Verification items for the finished model (mm, model axes). A direction names the side the tool comes from. Coordinates: 2 decimals unless noted, no trailing zeros. Write each loop counter-clockwise with the first axis right and the second up, starting at its lowest first coordinate (ties: lowest second). Pieces come first, ordered by that corner, then holes. Notation, with made-up numbers: (-22.75, 10) - (-16.75, 10) arc R13 cw to (-16.75, 29) - close; hole circle Ø2 at (2.25, -12.75). An arc over 180 degrees is marked (long way). Answer as CSV lines item,"result". Start each with the question number.
```python
from build123d import *

# Parameters (mm, degrees)
SKETCH1_W           = 90.48
SKETCH1_H           = 132.76
SKETCH1_W_2         = 85.48
SKETCH1_H_2         = 127.76
BOSS_EXTRUDE1_DEPTH = 16
SKETCH2_W           = 90.48
SKETCH2_H           = 132.76
BOSS_EXTRUDE2_DEPTH = 2.5
SKETCH3_R           = 7.5
BOSS_EXTRUDE3_DEPTH = 25
SKETCH4_R           = 7.5
SKETCH4_R_2         = 5
BOSS_EXTRUDE4_DEPTH = 25
SKETCH5_R           = 11
SKETCH5_R_2         = 5
BOSS_EXTRUDE5_DEPTH = 5
SKETCH7_R           = 5
CUT_EXTRUDE2_DEPTH  = 20
CUT_EXTRUDE3_REACH  = 134.76
SKETCH8_R           = 1.75
BOSS_EXTRUDE6_DEPTH = 5
SKETCH10_W          = 65.48
SKETCH10_H          = 107.76
CUT_EXTRUDE4_DEPTH  = 5.25


with BuildPart() as part:
    # Sketch1 → Boss-Extrude1 (new body)
    with BuildSketch(Plane(origin=(0, 0, 0), x_dir=(1, 0, 0), z_dir=(0, 1, 0))):
        Rectangle(SKETCH1_W, SKETCH1_H)
        Rectangle(SKETCH1_W_2, SKETCH1_H_2, mode=Mode.SUBTRACT)
    extrude(amount=BOSS_EXTRUDE1_DEPTH)

    # Sketch2 → Boss-Extrude2 (add)
    with BuildSketch(Plane.XZ):
        Rectangle(SKETCH2_W, SKETCH2_H)
    extrude(amount=BOSS_EXTRUDE2_DEPTH)

    # Sketch3 → Boss-Extrude3 (add)
    with BuildSketch(Plane(origin=(0, 0, -66.38), x_dir=(-1, 0, 0), z_dir=(0, 0, -1))):
        with BuildLine():
            Line((-45.24, 16), (-60, 16))
            ThreePointArc((-60, 16), (-69.25, 6.75), (-60, -2.5))
            Line((-60, -2.5), (-45.24, -2.5))
            Line((-45.24, -2.5), (-45.24, 16))
        make_face()
        with Locations((-60, 6.75)):
            Circle(SKETCH3_R, mode=Mode.SUBTRACT)
    boss_extrude3 = extrude(amount=-BOSS_EXTRUDE3_DEPTH)

    # Mirror1: Boss-Extrude3 across plane
    add(boss_extrude3.mirror(Plane(origin=(0, 0, 0), x_dir=(0, 0, 1), z_dir=(1, 0, 0))))

    # Sketch4 → Boss-Extrude4 (add)
    with BuildSketch(Plane(origin=(0, 0, -66.38), x_dir=(-1, 0, 0), z_dir=(0, 0, -1))):
        with Locations((60, 6.75)):
            Circle(SKETCH4_R)
        with Locations((60, 6.75)):
            Circle(SKETCH4_R_2, mode=Mode.SUBTRACT)
    extrude(amount=-BOSS_EXTRUDE4_DEPTH)

    # Sketch5 → Boss-Extrude5 (add)
    with BuildSketch(Plane(origin=(0, 0, -66.38), x_dir=(-1, 0, 0), z_dir=(0, 0, -1))):
        with Locations((60, 6.75)):
            Circle(SKETCH5_R)
        with Locations((60, 6.75)):
            Circle(SKETCH5_R_2, mode=Mode.SUBTRACT)
    extrude(amount=-BOSS_EXTRUDE5_DEPTH)

    # Sketch7 → Cut-Extrude2 (cut)
    with BuildSketch(Plane.XY.offset(-41.38)):
        with Locations((-60, 6.75)):
            Circle(SKETCH7_R)
        with BuildLine():
            Line((-45.24, -2.5), (-60, -2.5))
            ThreePointArc((-60, -2.5), (-69.25, 6.75), (-60, 16))
            Line((-60, 16), (-45.24, 16))
            Line((-45.24, 16), (-45.24, 8.25))
            Line((-45.24, 8.25), (-54.190524981, 8.25))
            ThreePointArc((-54.190524981, 8.25), (-66, 6.75), (-54.190524981, 5.25))
            Line((-54.190524981, 5.25), (-45.24, 5.25))
            Line((-45.24, 5.25), (-45.24, -2.5))
        make_face()
    extrude(amount=-CUT_EXTRUDE2_DEPTH, mode=Mode.SUBTRACT)

    # Sketch8 → Cut-Extrude3 (cut, up to next)
    with BuildSketch(Plane(origin=(0, 0, -66.38), x_dir=(-1, 0, 0), z_dir=(0, 0, -1)), mode=Mode.PRIVATE) as cut_extrude3_sk1:
        with Locations((60, 14.75)):
            Circle(SKETCH8_R)
    cut_extrude3_tool1 = extrude(cut_extrude3_sk1.sketch, amount=-CUT_EXTRUDE3_REACH, mode=Mode.PRIVATE) & part.part
    add(cut_extrude3_tool1.solids().sort_by_distance((-60, 14.75, -66.38))[0], mode=Mode.SUBTRACT)
    # Sketch8 → Cut-Extrude3 (cut, up to next)
    with BuildSketch(Plane(origin=(0, 0, -66.38), x_dir=(-1, 0, 0), z_dir=(0, 0, -1)), mode=Mode.PRIVATE) as cut_extrude3_sk2:
        with Locations((68, 6.75)):
            Circle(SKETCH8_R)
    cut_extrude3_tool2 = extrude(cut_extrude3_sk2.sketch, amount=-CUT_EXTRUDE3_REACH, mode=Mode.PRIVATE) & part.part
    add(cut_extrude3_tool2.solids().sort_by_distance((-68, 6.75, -66.38))[0], mode=Mode.SUBTRACT)
    # Sketch8 → Cut-Extrude3 (cut, up to next)
    with BuildSketch(Plane(origin=(0, 0, -66.38), x_dir=(-1, 0, 0), z_dir=(0, 0, -1)), mode=Mode.PRIVATE) as cut_extrude3_sk3:
        with Locations((60, -1.25)):
            Circle(SKETCH8_R)
    cut_extrude3_tool3 = extrude(cut_extrude3_sk3.sketch, amount=-CUT_EXTRUDE3_REACH, mode=Mode.PRIVATE) & part.part
    add(cut_extrude3_tool3.solids().sort_by_distance((-60, -1.25, -66.38))[0], mode=Mode.SUBTRACT)

    # Sketch9 → Boss-Extrude6 (add)
    with BuildSketch(Plane(origin=(0, 16, 0), x_dir=(1, 0, 0), z_dir=(0, 1, 0))):
        Polygon((33.74, 63.88), (42.74, 54.88), (42.74, 63.88), align=None)
        Polygon((-42.74, 54.88), (-33.74, 63.88), (-42.74, 63.88), align=None)
    extrude(amount=-BOSS_EXTRUDE6_DEPTH)

    # Sketch10 → Cut-Extrude4 (cut, through all)
    with BuildSketch(Plane(origin=(0, 0, 0), x_dir=(1, 0, 0), z_dir=(0, 1, 0))):
        Rectangle(SKETCH10_W, SKETCH10_H)
    extrude(amount=-CUT_EXTRUDE4_DEPTH, mode=Mode.SUBTRACT)


solid = part.part
```
1. Depth check by flat-ended pin: P1, Ø12, axis at x = -29.5, z = 4, coming from the -Y side; P2, Ø3.5, axis at x = -58, y = 9.5, coming from the +Z side; P3, Ø0.8, axis at y = -1.5, z = -25.5, coming from the +X side. Enter the tip coordinate at first touch or a pass-through.
2. Draft check along X on faces 5 (the face through (-70.995, 6.42, -63.915)), 6 (the face through (-65.995, 6.993, -51.24)), 7 (the face through (-50, 8.25, -51)), 8 (the face through (45, 16, -25)). Enter one of: pulls with the +X half, pulls with the -X half, needs draft (parallel to the pull), parting line crosses it, or undercut.
3. Cross-section at C-C (x = -68). Record the cut outline in (y, z), and give its area (3 significant figures).
4. Cross-section at A-A (x = 14). Record the cut outline in (y, z), and give its area (4 significant figures).
5. Access from +Z, -Z, +X, -X, +Y, -Y to the whole of each face (thin tool, end or side, straight path). Record for faces 1 (the face through (-54.8, 7.2, -41.38)), 2 (the face through (38.18, 13.54, -59.44)), 3 (the face through (-1, 8, -63.88)), 4 (the face through (52, 7, -41.38)).
6. Cross-section at B-B (z = 31.5). Record the cut outline in (x, y), and give its area (4 significant figures).
7. Scan lines: line 1 along Y through (x, z) = (-60, -65.2); line 2 along X through (y, z) = (9.75, 38); line 3 along X through (y, z) = (-1.25, 9.5). Record each from-to range of solid material in increasing order. Write a range as from..to.
Completed:
1,P1,"stops at y = -2.5"
1,P2,"stops at z = -41.38"
1,P3,"stops at x = 45.24"
2,face 5,"parting line crosses it"
2,face 6,"undercut"
2,face 7,"undercut"
2,face 8,"needs draft"
3,outline,"(-0.8, -66.38) - (5, -66.38) - (5, -61.38) - (-0.8, -61.38) - close; (8.5, -66.38) - (14.3, -66.38) - (14.3, -61.38) - (8.5, -61.38) - close"
3,area,"58.0 mm2"
4,outline,"(-2.5, -66.38) - (16, -66.38) - (16, -63.88) - (0, -63.88) - (0, -53.88) - (-2.5, -53.88) - close; (-2.5, 53.88) - (0, 53.88) - (0, 63.88) - (16, 63.88) - (16, 66.38) - (-2.5, 66.38) - close"
4,area,"142.5 mm2"
5,face 1,"+Z, -X, +Y, -Y"
5,face 2,"+Y"
5,face 3,"none"
5,face 4,"+Z, +X, +Y, -Y"
6,outline,"(-45.24, -2.5) - (-32.74, -2.5) - (-32.74, 0) - (-42.74, 0) - (-42.74, 16) - (-45.24, 16) - close; (32.74, -2.5) - (45.24, -2.5) - (45.24, 16) - (42.74, 16) - (42.74, 0) - (32.74, 0) - close"
6,area,"142.5 mm2"
7,line 1,"y = -4.25..-3, 0.5..1.75, 11.75..13, 16.5..17.75"
7,line 2,"x = -45.24..-42.74, 42.74..45.24"
7,line 3,"x = -45.24..-32.74, 32.74..45.24"
